```python
from build123d import *

# Parameters (mm, degrees)
F0_R          = 17
F0_R_2        = 16
F1_DEPTH      = 150
F2_R          = 16
F2_R_2        = 15
F3_DEPTH      = 20
F3_DEPTH_BACK = 20
F4_SIZE2      = 19.0942296485
F4_SIZE       = 0.5


with BuildPart() as f1:
    # F0 (on Top) → F1 (new body)
    with BuildSketch(Plane.XY):
        Circle(F0_R)
        Circle(F0_R_2, mode=Mode.SUBTRACT)
    extrude(amount=F1_DEPTH)

    # F2 (on face) → F3 (join, two sides)
    with BuildSketch(Plane.XY.offset(150)) as f3_sk:
        Circle(F2_R)
        Circle(F2_R_2, mode=Mode.SUBTRACT)
    extrude(amount=F3_DEPTH)
    extrude(f3_sk.sketch, amount=-F3_DEPTH_BACK)

    # F4
    f4_edges = [f1.edges().sort_by_distance(p)[0] for p in [
        (-16, 0, 170),
    ]]
    f4_side = f1.faces().sort_by_distance((-15.547452, 0, 170))[0]
    chamfer(f4_edges, length=F4_SIZE, length2=F4_SIZE2, reference=f4_side)


solid = f1.part
```
Check sheet for the modelled part. Datum: model origin and axes. Units: mm. A direction names the side the tool comes from. Give positions to 0.01 mm unless a question says otherwise; leave off trailing zeros. Order: outer loops, then holes, each group sorted by start corner. A loop starts at its lowest first (then second) coordinate and runs counter-clockwise, first axis right, second up. Notation, with made-up numbers: M -30.5,66.5 L -4.5,66.5 A32 cw -4.5,100.5 Z; hole C -39,3 d8. An arc over 180 degrees is marked long. Answer in a Markdown table with one row per item. Add a question column.
Q1. Thickness scan on L1, parallel to Y at x = 0, z = 152; L2, parallel to Y at x = 0, z = 77; L3, parallel to Z at x = -11, y = -12. Record the ranges inside material, lowest first.
Q2. Sectioned sample at D-D, the plane z = 62. Record the boundary of the cut face in (x, y).
Q3. Sectioned sample at C-C, the plane z = 133. Record the boundary of the cut face in (x, y), and give its area (3 significant figures).
Q4. Access from +Z, -Z, +X, -X, +Y, -Y to the whole of each face (thin tool, end or side, straight path). Record for faces 1 (the cylindrical face through (-3.47, -15.62, 64.09)), 2 (the conical face through (15.026, 4.732, 160.319)), 3 (the flat face through (13, -10, 0)).
Q5. Release check for a two-part mould opening along X. For faces 4 (the cylindrical face through (9.139, 14.334, 73.95)), 5 (the cylindrical face through (-14.985, 0.66, 149.72)), 6 (the flat face through (-8, 13, 170)) record: released by +X, released by -X, zero draft, split by the parting line, or undercut.
Q6. Sectioned sample at A-A, the plane x = 0. Record the boundary of the cut face in (y, z), and give its area (3 significant figures).
Q7. Gauge pin test, flat ends, axial feed: pin 1 Ø3 at (x, z) = (-8, 19) entering from +Y; pin 2 Ø8 at (x, z) = (12, 131.5) entering from +Y; pin 3 Ø8 at (y, z) = (13, 42) entering from -X; pin 4 Ø8 at (x, y) = (-13, 4.5) entering from -Z. Record the tip position at first contact, or that the pin passes through.
Verdict:
| question | item | result |
|---|---|---|
| 1 | L1 | -15.97 to -15, 15 to 15.97 |
| 1 | L2 | -17 to -16, 16 to 17 |
| 1 | L3 | 0 to 150 |
| 2 | outline | C 0,0 d34; hole C 0,0 d32 |
| 3 | outline | C 0,0 d34; hole C 0,0 d30 |
| 3 | area | 201 mm² |
| 4 | face 1 | -Z |
| 4 | face 2 | +Z |
| 4 | face 3 | -Z, +X, -X, +Y, -Y |
| 5 | face 4 | split by the parting line |
| 5 | face 5 | undercut |
| 5 | face 6 | zero draft |
| 6 | outline | M -17,0 L -16,0 L -16,130 L -15,130 L -15,170 L -15.5,170 L -16,150.91 L -16,150 L -17,150 Z; M 15,130 L 16,130 L 16,0 L 17,0 L 17,150 L 16,150 L 16,150.91 L 15.5,170 L 15,170 Z |
| 6 | area | 370 mm² |
| 7 | pin 1 | y = 15.71 |
| 7 | pin 2 | y = 15 |
| 7 | pin 3 | x = -14.42 |
| 7 | pin 4 | z = 0 |
